Check sheet for the modelled part. Datum: model origin and axes. Units: mm. A direction names the side the tool comes from. Round coordinates to 2 decimals unless told otherwise and drop trailing zeros. Loops run counter-clockwise (first coordinate to the right, second up) from the corner with the lowest first, then second, coordinate; pieces in that order, holes last. Notation, with made-up numbers: (60, 71) - (105, 71) arc R21 cw to (105, 92) - close; hole circle Ø9 at (50.5, -9). An arc over 180 degrees is marked (long way). Put each result on its own line as item: value.
```python
from build123d import *

# Parameters (mm, degrees)
SKETCH_1_R      = 1.5
SKETCH_1_R_2    = 3
EXTRUDE_1_DEPTH = 1


with BuildPart() as part:
    # 草图1 → 凸台-拉伸1 (new body)
    with BuildSketch(Plane(origin=(0, 0, 0), x_dir=(1, 0, 0), z_dir=(0, 1, 0))):
        with BuildLine():
            Line((-25.835275078, 96.418559218), (-4.937952664, 18.428690227))
            ThreePointArc((-4.937952664, 18.428690227), (-5.142265363, 14.699078916), (-7.513455335, 11.81304317))
            ThreePointArc((-7.513455335, 11.81304317), (-9.899494937, -9.899494937), (11.81304317, -7.513455335))
            ThreePointArc((11.81304317, -7.513455335), (14.699078916, -5.142265363), (18.428690227, -4.937952664))
            Line((18.428690227, -4.937952664), (96.418559218, -25.835275078))
            ThreePointArc((96.418559218, -25.835275078), (101.126076798, -25.143491075), (103.849761898, -21.242103327))
            ThreePointArc((103.849761898, -21.242103327), (74.953318806, 74.953318806), (-21.242103327, 103.849761898))
            ThreePointArc((-21.242103327, 103.849761898), (-25.143491075, 101.126076798), (-25.835275078, 96.418559218))
        make_face()
        with Locations(Location((0, 9.5, 0), (0, 0, 270))):
            Circle(SKETCH_1_R, mode=Mode.SUBTRACT)
        with Locations(Location((9.5, 0, 0), (0, 0, 270))):
            Circle(SKETCH_1_R, mode=Mode.SUBTRACT)
        with Locations(Location((0, -9.5, 0), (0, 0, 270))):
            Circle(SKETCH_1_R, mode=Mode.SUBTRACT)
        with Locations(Location((-9.5, 0, 0), (0, 0, 270))):
            Circle(SKETCH_1_R, mode=Mode.SUBTRACT)
        with Locations(Location((0, 0, 0), (0, 0, 270))):
            Circle(SKETCH_1_R_2, mode=Mode.SUBTRACT)
        with Locations(Location((72.124891681, 72.124891681, 0), (0, 0, 270))):
            Circle(SKETCH_1_R, mode=Mode.SUBTRACT)
        with Locations(Location((99.582192726, -22.076840622, 0), (0, 0, 270))):
            Circle(SKETCH_1_R, mode=Mode.SUBTRACT)
        with Locations(Location((-22.076840622, 99.582192726, 0), (0, 0, 90))):
            Circle(SKETCH_1_R, mode=Mode.SUBTRACT)
        with BuildLine():
            Line((67.963499444, 64.427965538), (14.219339812, 10.683805906))
            ThreePointArc((14.219339812, 10.683805906), (12.666425541, 4.888250948), (16.909066229, 0.645610261))
            Line((16.909066229, 0.645610261), (91.467293555, -19.33220654))
            ThreePointArc((91.467293555, -19.33220654), (96.31960421, -18.54803697), (98.9576679, -14.400693173))
            ThreePointArc((98.9576679, -14.400693173), (96.237907867, 27.171034013), (76.815042692, 64.026941331))
            ThreePointArc((76.815042692, 64.026941331), (72.477694994, 66.17917653), (67.963499444, 64.427965538))
        make_face(mode=Mode.SUBTRACT)
        with BuildLine():
            Line((64.427965538, 67.963499444), (10.683805906, 14.219339812))
            ThreePointArc((10.683805906, 14.219339812), (4.888250948, 12.666425541), (0.645610261, 16.909066229))
            Line((0.645610261, 16.909066229), (-19.33220654, 91.467293555))
            ThreePointArc((-19.33220654, 91.467293555), (-18.54803697, 96.31960421), (-14.400693173, 98.9576679))
            ThreePointArc((-14.400693173, 98.9576679), (27.171034013, 96.237907867), (64.026941331, 76.815042692))
            ThreePointArc((64.026941331, 76.815042692), (66.17917653, 72.477694994), (64.427965538, 67.963499444))
        make_face(mode=Mode.SUBTRACT)
    extrude(amount=EXTRUDE_1_DEPTH)


solid = part.part
```
Item 1: Tool access check on faces 4 (the cylindrical face through (12.644, 0.493, -4.973)), 5 (the flat face through (56.88, 0.49, 15.24)), 6 (the flat face through (40, 1, -40)). Record the directions out of +Z, -Z, +X, -X, +Y, -Y that give a thin tool (end or side, any length) a straight path to the whole face; none if there is none.
Filled sheet:
face 4: +Y, -Y
face 5: +Z, +Y, -Y
face 6: +Z, -Z, +X, -X, +Y
Item 2: Section check D-D on y = 0.55. Count the separate pieces of the cut face and the enclosed holes in it, then the cut area to 3 significant figures.
Filled sheet:
separate pieces: 1
enclosed holes: 10
area: 3,160 mm²
Item 3: Section check B-B on x = 46.5. Enter the section's corners in (y, z).
Filled sheet:
outline: (0, -95.26) - (1, -95.26) - (1, -88.53) - (0, -88.53) - close; (0, -50.04) - (1, -50.04) - (1, -42.96) - (0, -42.96) - close; (0, 7.28) - (1, 7.28) - (1, 12.46) - (0, 12.46) - close
Item 4: Thickness scan on line 1 (Z direction, x = 31, y = 0.4); line 2 (X direction, y = 0.3, z = -47); line 3 (X direction, y = 0.95, z = -33.5). Record the ranges inside material, lowest first. Write a range as from..to.
Filled sheet:
line 1: -101.37..-95.07, -34.54..-27.46, 3.13..8.31
line 2: -12.59..-7.42, 43.46..50.54, 88.27..95.01
line 3: -8.98..-3.8, 29.96..37.04, 94.22..100.57
Item 5: Release check for a two-part mould opening along Z. For faces 1 (the cylindrical face through (-25.11, 0.49, -101.18)), 2 (the flat face through (-9.203, 0.493, -53.666)), 3 (the cylindrical face through (101.07, 0.49, 25.18)) record: +Z half, -Z half, draft (parallel to the pull), parting line (faces both ways), or undercut.
Filled sheet:
face 1: parting line
face 2: undercut
face 3: +Z half
Item 6: Section check A-A on z = 9.5. Enter the section's corners in (x, y).
Filled sheet:
outline: (-10.28, 0) - (-1.5, 0) - (-1.5, 1) - (-10.28, 1) - close; (1.5, 0) - (10.28, 0) - (10.28, 1) - (1.5, 1) - close; (35.45, 0) - (54.77, 0) - (54.77, 1) - (35.45, 1) - close; (99.55, 0) - (105.57, 0) - (105.57, 1) - (99.55, 1) - close
Item 7: Section check C-C on z = -83. Enter the section's corners in (x, y).
Filled sheet:
outline: (-22.24, 0) - (-17.06, 0) - (-17.06, 1) - (-22.24, 1) - close; (55.78, 0) - (65.93, 0) - (65.93, 1) - (55.78, 1) - close
